Verification items for the finished model (mm, model axes). Face numbers are marked on the shaded views. A direction names the side the tool comes from. Give positions to 0.01 mm unless a question says otherwise; leave off trailing zeros.
(1) Gauge pin test, flat ends, axial feed: pin 1 (1 mm diameter, centred on y = 0, z = -2, fed in from -X); pin 2 (1.5 mm diameter, centred on x = -6.5, y = -0.5, fed in from +Z); pin 3 (1 mm diameter, centred on x = -5, y = 2.5, fed in from +Z); pin 4 (1.5 mm diameter, centred on x = -1, z = -2.5, fed in from -Y). Record the tip position at first contact, or that the pin passes through.
(2) Scan lines: L1, parallel to Y at x = -1.95, z = 0; L2, parallel to Y at x = -1.5, z = 2. Record each from-to range of solid material in increasing order.
(3) Access from +Z, -Z, +X, -X, +Y, -Y to the whole of each face (thin tool, end or side, straight path). Record for the marked faces 5, 6, 7 and 8.
(4) Mould release check, pull along Y, two halves, no side actions. Record for the marked faces 1, 2, 3 and 4: pulls with the +Y half, pulls with the -Y half, needs draft (parallel to the pull), parting line crosses it, or undercut.
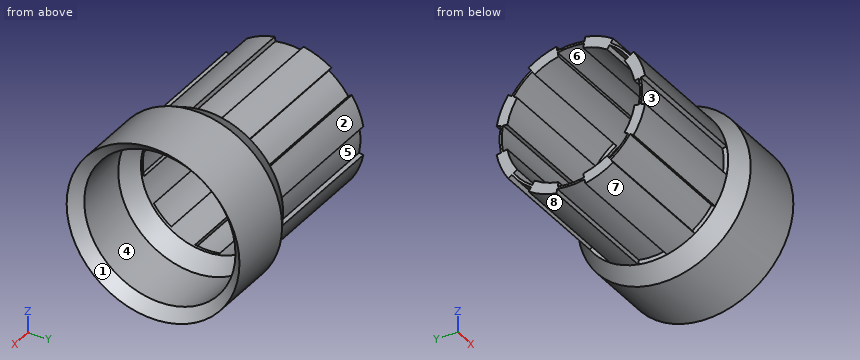
```python
from build123d import *

# Parameters (mm, degrees)
CUT_EXTRUDE1_DEPTH = 6
CIRPATTERN1_COUNT  = 8
CHAMFER1_SIZE      = 0.5


with BuildPart() as part:
    # Sketch2 → Revolve1 (revolve)
    with BuildSketch(Plane.XY):
        Polygon((-10, 3), (-10, 3.5), (-4, 3.5), (-3.133974596, 4), (0, 4), (0, 3.5), (-3, 3.5), (-3.866025404, 3), align=None)
    revolve(axis=Axis((-10, 0, 0), (-1, 0, 0)))

    # Sketch3 → Cut-Extrude1 (cut)
    with BuildSketch(Plane.ZY.offset(10)):
        with BuildLine():
            Line((0.572426986, 2.94488155), (0.610588785, 3.141206987))
            ThreePointArc((0.610588785, 3.141206987), (0, 3.2), (-0.610588785, 3.141206987))
            Line((-0.610588785, 3.141206987), (-0.572426986, 2.94488155))
            ThreePointArc((-0.572426986, 2.94488155), (0, 3), (0.572426986, 2.94488155))
        make_face()
        with BuildLine():
            Line((-0.629669685, 3.239369705), (-0.667831484, 3.435695142))
            ThreePointArc((-0.667831484, 3.435695142), (0, 3.5), (0.667831484, 3.435695142))
            Line((0.667831484, 3.435695142), (0.629669685, 3.239369705))
            ThreePointArc((0.629669685, 3.239369705), (0, 3.3), (-0.629669685, 3.239369705))
        make_face()
    cut_extrude1 = extrude(amount=-CUT_EXTRUDE1_DEPTH, mode=Mode.SUBTRACT)

    # CirPattern1: Cut-Extrude1 ×8 about axis
    cirpattern1_axis = Axis((0, 0, 0), (1, 0, 0))
    for i in range(1, CIRPATTERN1_COUNT):
        add(cut_extrude1.rotate(cirpattern1_axis, i * 360 / CIRPATTERN1_COUNT), mode=Mode.SUBTRACT)

    # Chamfer1
    chamfer1_edges = [part.edges().sort_by_distance(p)[0] for p in [
        (0, -3.5, 0),
    ]]
    chamfer(chamfer1_edges, length=CHAMFER1_SIZE - 0.0001)  # a hair under: the kernel refuses the full size


solid = part.part
```
Ans:
1. pin 1: passes through
1. pin 2: stops at z = 3.44
1. pin 3: stops at z = 2.62
1. pin 4: stops at y = -3.6
2. L1: y = -4 to -3.5, 3.5 to 4
2. L2: y = -3.46 to -2.87, 2.87 to 3.46
3. face 5: -X, +Y
3. face 6: -X
3. face 7: -Z, -X, -Y
3. face 8: -Z, -X, +Y
4. face 1: undercut
4. face 2: pulls with the +Y half
4. face 3: pulls with the -Y half
4. face 4: undercut
